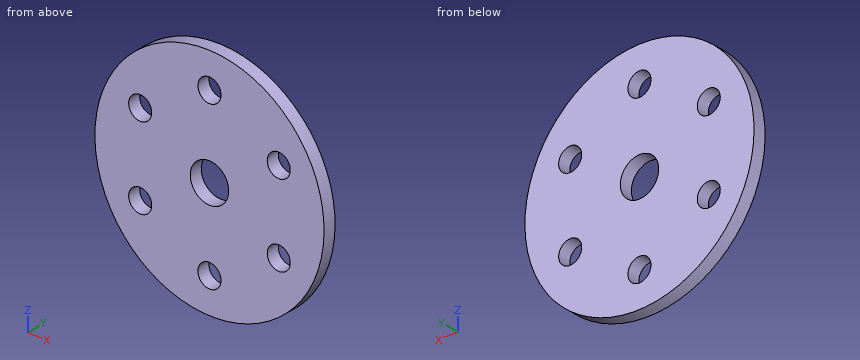
```python
from build123d import *

# Parameters (mm, degrees)
SKETCH1_R            = 17.9
SKETCH1_R_2          = 3
BOSS_EXTRUDE1_DEPTH  = 2
M3_CLEARANCE_HOLE1_D = 3.6


with BuildPart() as part:
    # Sketch1 → Boss-Extrude1 (new body)
    with BuildSketch(Plane(origin=(0, 0, 0), x_dir=(1, 0, 0), z_dir=(0, 1, 0))):
        with Locations(Location((0, 0, 0), (0, 0, 270))):
            Circle(SKETCH1_R)
        with Locations(Location((0, 0, 0), (0, 0, 270))):
            Circle(SKETCH1_R_2, mode=Mode.SUBTRACT)
    extrude(amount=BOSS_EXTRUDE1_DEPTH)

    # M3 Clearance Hole1 (through all)
    with Locations(Plane(origin=(0, 2, 0), x_dir=(1, 0, 0), z_dir=(0, 1, 0))):
        with Locations((0, 12.5), (-10.825317547, 6.25), (-10.825317547, -6.25), (0, -12.5), (10.825317547, -6.25), (10.825317547, 6.25)):
            Hole(M3_CLEARANCE_HOLE1_D / 2)


solid = part.part
```
CAD build for the part. Positions are in the model's coordinates, mm. Coordinates: 2 decimals unless noted, no trailing zeros. Write each loop counter-clockwise with the first axis right and the second up, starting at its lowest first coordinate (ties: lowest second). Pieces come first, ordered by that corner, then holes. Notation, with made-up numbers: (38.25, 24.25) -> (59.25, 24.25) arc R22 ccw to (59.25, 50.25) -> close; hole circle Ø2 at (62.5, 89.5). An arc over 180 degrees is marked (long way). Return JSON: item names as keys, results as strings. Group by question number.
Q1. Cut at B-B, the plane z = 0. Give the cut face in (x, y), then the cut area to 3 significant figures.
Q2. Cut at A-A, the plane y = 1.05. Give the cut face in (x, z), then the cut area to 3 significant figures.
Q3. Drill centre lines: line 1 (X direction, y = 1.3, z = 6); line 2 (X direction, y = 0.7, z = 0); line 3 (X direction, y = 0.5, z = -6.25). Where is each one in solid material? Low to high.
Q4. Cut at D-D, the plane z = -12.5. Give the cut face in (x, y).
Q5. Cut at C-C, the plane z = 6.25. Give the cut face in (x, y).
Returned:
{
 "1": {"outline": "(-17.9, 0) -> (-3, 0) -> (-3, 2) -> (-17.9, 2) -> close; (3, 0) -> (17.9, 0) -> (17.9, 2) -> (3, 2) -> close", "area": "59.6 mm2"},
 "2": {"outline": "circle Ø35.8 at (0, 0); hole circle Ø3.6 at (-10.83, -6.25); hole circle Ø3.6 at (-10.83, 6.25); hole circle Ø6 at (0, 0); hole circle Ø3.6 at (0, -12.5); hole circle Ø3.6 at (0, 12.5); hole circle Ø3.6 at (10.83, -6.25); hole circle Ø3.6 at (10.83, 6.25)", "area": "917 mm2"},
 "3": {"line 1": "x = -16.86 to -12.61, -9.04 to 9.04, 12.61 to 16.86", "line 2": "x = -17.9 to -3, 3 to 17.9", "line 3": "x = -16.77 to -12.63, -9.03 to 9.03, 12.63 to 16.77"},
 "4": {"outline": "(-12.81, 0) -> (-1.8, 0) -> (-1.8, 2) -> (-12.81, 2) -> close; (1.8, 0) -> (12.81, 0) -> (12.81, 2) -> (1.8, 2) -> close"},
 "5": {"outline": "(-16.77, 0) -> (-12.63, 0) -> (-12.63, 2) -> (-16.77, 2) -> close; (-9.03, 0) -> (9.03, 0) -> (9.03, 2) -> (-9.03, 2) -> close; (12.63, 0) -> (16.77, 0) -> (16.77, 2) -> (12.63, 2) -> close"}
}
